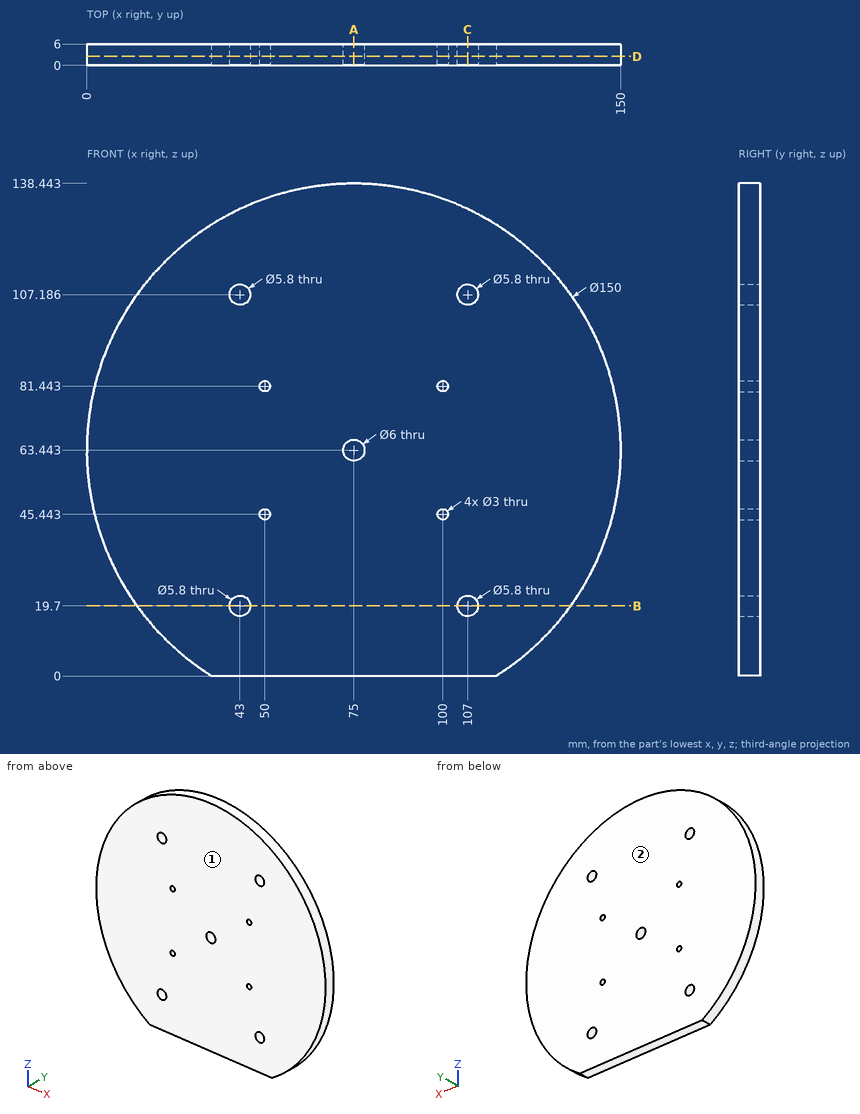
Source: three-view drawing plus pictorial views. Frame: mm from the lowest corner of the part. Coordinates: 2 decimals unless noted, no trailing zeros. Order: outer loops, then holes, each group sorted by start corner. A loop starts at its lowest first (then second) coordinate and runs counter-clockwise, first axis right, second up. Notation, with made-up numbers: M 62.25,-37.75 L 120.25,-37.75 A21 cw 120.25,-29.75 Z; hole C 83,-5.75 d11. An arc over 180 degrees is marked long. One line per question, with ' | ' between items.
Item 1: Ray query, line 1 along Z through (x, y) = (75, 4.4); line 2 along Z through (x, y) = (100, 2.7); line 3 along Z through (x, y) = (107, 1.4) (1 decimal). Return the intervals inside material, ascending.
Geometry results:
line 1: z = 0 to 60.44, 66.44 to 138.44 | line 2: z = 0 to 43.94, 46.94 to 79.94, 82.94 to 134.15 | line 3: z = 0 to 16.8, 22.6 to 104.3, 110.1 to 131.3
Item 2: Section A-A (x = 75). Output: boundary loops of the cut face in (y, z), then the cut area to 3 significant figures.
Geometry results:
outline: M 0,0 L 6,0 L 6,60.44 L 0,60.44 Z; M 0,66.44 L 6,66.44 L 6,138.44 L 0,138.44 Z | area: 795 mm^2
Item 3: Section C-C (x = 107). Output: boundary loops of the cut face in (y, z).
Geometry results:
outline: M 0,0 L 6,0 L 6,16.8 L 0,16.8 Z; M 0,22.6 L 6,22.6 L 6,104.29 L 0,104.29 Z; M 0,110.09 L 6,110.09 L 6,131.27 L 0,131.27 Z
Item 4: Pin query (flat end, axial travel): pin 1 (1.5 mm diameter, centred on x = 103, y = 5, fed in from +Z); pin 2 (2 mm diameter, centred on x = 85.5, y = 5, fed in from +Z). Return the tip coordinate at first contact, or that it passes through.
Geometry results:
pin 1: stops at z = 133.32 | pin 2: stops at z = 137.84
Item 5: Section B-B (z = 19.7). Output: boundary loops of the cut face in (x, y).
Geometry results:
outline: M 14.08,0 L 40.1,0 L 40.1,6 L 14.08,6 Z; M 45.9,0 L 104.1,0 L 104.1,6 L 45.9,6 Z; M 109.9,0 L 135.92,0 L 135.92,6 L 109.9,6 Z
Item 6: Section D-D (y = 2.55). Give the number of separate pieces and of enclosed holes in the cut face, then the cut area to 3 significant figures.
Geometry results:
separate pieces: 1 | enclosed holes: 9 | area: 16,900 mm^2
Item 7: Draft query along Y for the marked faces 1 and 2. Return one class per face: released by +Y, released by -Y, zero draft, split by the parting line, or undercut.
Geometry results:
face 1: released by -Y | face 2: released by +Y
